from build123d import *

# Parameters (mm, degrees)
SKETCH1_W           = 233.2
SKETCH1_H           = 100
SKETCH1_R           = 1.55
BOSS_EXTRUDE1_DEPTH = 6.35
FILLET1_R           = 5
SKETCH2_R           = 1.55
CUT_EXTRUDE1_DEPTH  = 6.35
SKETCH3_W           = 10
SKETCH3_H           = 12.7
BOSS_EXTRUDE2_DEPTH = 6.35
FILLET2_R           = 5
FILLET3_R           = 10
FILLET4_R           = 2
FILLET5_R           = 20
FILLET6_R           = 5
CUT_EXTRUDE2_DEPTH  = 10
SKETCH5_W           = 120
SKETCH5_H           = 40
CUT_EXTRUDE4_DEPTH  = 10
SKETCH6_R           = 1.5
CUT_EXTRUDE5_DEPTH  = 10
FILLET7_R           = 10
SKETCH7_W           = 25
SKETCH7_H           = 35
CUT_EXTRUDE6_DEPTH  = 10
FILLET9_R           = 10
SKETCH8_R           = 1.5
CUT_EXTRUDE7_DEPTH  = 10
BOSS_EXTRUDE3_START = -6.35
BOSS_EXTRUDE3_DEPTH = 6.35
FILLET10_R          = 5
BOSS_EXTRUDE4_START = -6.35
BOSS_EXTRUDE4_DEPTH = 6.35
FILLET11_R          = 3
FILLET12_R          = 3
CUT_EXTRUDE8_DEPTH  = 10
FILLET13_R          = 3
CUT_EXTRUDE9_DEPTH  = 10
SKETCH13_R          = 1.55
CUT_EXTRUDE10_DEPTH = 10
SKETCH14_R          = 1.5
CUT_EXTRUDE11_DEPTH = 10
BOSS_EXTRUDE5_START = -6.35
BOSS_EXTRUDE5_DEPTH = 6.35
FILLET14_R          = 10
SKETCH15_R          = 1.55
CUT_EXTRUDE12_DEPTH = 254.816001269


# Read off the part's stored shape, not the designer's step: Boss-Extrude5
with BuildPart() as part:
    # Sketch1 → Boss-Extrude1 (new body)
    with BuildSketch(Plane.XY):
        with Locations((116.6, -50)):
            Rectangle(SKETCH1_W, SKETCH1_H)
        with Locations((7.5, -10)):
            Circle(SKETCH1_R, mode=Mode.SUBTRACT)
        with Locations((225.7, -10)):
            Circle(SKETCH1_R, mode=Mode.SUBTRACT)
        with Locations((7.5, -90)):
            Circle(SKETCH1_R, mode=Mode.SUBTRACT)
        with Locations((225.7, -90)):
            Circle(SKETCH1_R, mode=Mode.SUBTRACT)
        with Locations((27.5, -10)):
            Circle(SKETCH1_R, mode=Mode.SUBTRACT)
        with Locations((205.7, -10)):
            Circle(SKETCH1_R, mode=Mode.SUBTRACT)
        with Locations((134.6, -10)):
            Circle(SKETCH1_R, mode=Mode.SUBTRACT)
        with Locations((98.6, -10)):
            Circle(SKETCH1_R, mode=Mode.SUBTRACT)
    extrude(amount=BOSS_EXTRUDE1_DEPTH)

    # Fillet1
    fillet1_edges = [part.edges().sort_by_distance(p)[0] for p in [
        (233.2, -100, 3.175),
        (0, -100, 3.175),
        (0, 0, 3.175),
        (233.2, 0, 3.175),
    ]]
    fillet(fillet1_edges, radius=FILLET1_R)

    # Sketch2 → Cut-Extrude1 (cut)
    with BuildSketch(Plane.XY.offset(6.35)):
        with Locations((45, -25)):
            Circle(SKETCH2_R)
        with Locations((45, -49)):
            Circle(SKETCH2_R)
        with Locations(Location((188.2, -49, 0), (0, 0, 180))):
            Circle(SKETCH2_R)
        with Locations(Location((188.2, -25, 0), (0, 0, 180))):
            Circle(SKETCH2_R)
    extrude(amount=-CUT_EXTRUDE1_DEPTH, mode=Mode.SUBTRACT)

    # Sketch3 → Boss-Extrude2 (add)
    with BuildSketch(Plane.XY.offset(6.35)):
        with Locations((125.723568259, 6.35)):
            Rectangle(SKETCH3_W, SKETCH3_H)
        Polygon((120.723568259, 16.7), (120.723568259, 12.7), (130.723568259, 12.7), (130.723568259, 24.7), (85.723568259, 24.7), (85.723568259, 12.7), (95.723568259, 12.7), (95.723568259, 16.7), align=None)
        Polygon((130.723568259, 12.7), (130.723568259, 0), (152.313568259, 0), (130.723568259, 24.7), align=None)
    extrude(amount=-BOSS_EXTRUDE2_DEPTH)

    # Fillet2
    fillet2_edges = [part.edges().sort_by_distance(p)[0] for p in [
        (85.723568259, 12.7, 3.175),
    ]]
    fillet(fillet2_edges, radius=FILLET2_R)

    # Fillet3
    fillet3_edges = [part.edges().sort_by_distance(p)[0] for p in [
        (120.723568259, 0, 3.175),
    ]]
    fillet(fillet3_edges, radius=FILLET3_R)

    # Fillet4
    fillet4_edges = [part.edges().sort_by_distance(p)[0] for p in [
        (85.723568259, 24.7, 3.175),
    ]]
    fillet(fillet4_edges, radius=FILLET4_R)

    # Fillet5
    fillet5_edges = [part.edges().sort_by_distance(p)[0] for p in [
        (130.723568259, 24.7, 3.175),
        (152.313568259, 0, 3.175),
    ]]
    fillet(fillet5_edges, radius=FILLET5_R)

    # Fillet6
    fillet6_edges = [part.edges().sort_by_distance(p)[0] for p in [
        (120.723568259, 16.7, 3.175),
    ]]
    fillet(fillet6_edges, radius=FILLET6_R)

    # Sketch4 → Cut-Extrude2 (cut)
    with BuildSketch(Plane(origin=(0, 0, 0), x_dir=(-1, 0, 0), z_dir=(0, 0, -1))):
        with BuildLine():
            Line((-110.723568259, 0), (-161.395157905, 0))
            ThreePointArc((-161.395157905, 0), (-153.126132222, 1.789475179), (-146.33682816, 6.837678575))
            Line((-146.33682816, 6.837678575), (-136.700308357, 17.862321425))
            ThreePointArc((-136.700308357, 17.862321425), (-129.911004296, 22.910524821), (-121.641978613, 24.7))
            Line((-121.641978613, 24.7), (-87.723568259, 24.7))
            ThreePointArc((-87.723568259, 24.7), (-86.309354696, 24.114213562), (-85.723568259, 22.7))
            Line((-85.723568259, 22.7), (-85.723568259, 17.7))
            ThreePointArc((-85.723568259, 17.7), (-87.188034353, 14.164466094), (-90.723568259, 12.7))
            Line((-90.723568259, 12.7), (-95.723568259, 12.7))
            Line((-95.723568259, 12.7), (-95.723568259, 16.7))
            Line((-95.723568259, 16.7), (-115.723568259, 16.7))
            ThreePointArc((-115.723568259, 16.7), (-119.259102165, 15.235533906), (-120.723568259, 11.7))
            Line((-120.723568259, 11.7), (-120.723568259, 10))
            ThreePointArc((-120.723568259, 10), (-117.794636071, 2.928932188), (-110.723568259, 0))
        make_face()
    extrude(amount=-CUT_EXTRUDE2_DEPTH, mode=Mode.SUBTRACT)

    # Sketch5 → Cut-Extrude4 (cut)
    with BuildSketch(Plane.XY.offset(6.35)):
        Polygon((56.6, -100), (56.6, -60), (26.6, -100), align=None)
        with Locations((116.6, -80)):
            Rectangle(SKETCH5_W, SKETCH5_H)
        Polygon((206.6, -100), (176.6, -60), (176.6, -100), align=None)
    extrude(amount=-CUT_EXTRUDE4_DEPTH, mode=Mode.SUBTRACT)

    # Sketch6 → Cut-Extrude5 (cut)
    with BuildSketch(Plane.XY.offset(6.35)):
        with Locations((71.6, -21.25)):
            Circle(SKETCH6_R)
        with Locations((161.6, -21.25)):
            Circle(SKETCH6_R)
        with Locations((161.6, -52.75)):
            Circle(SKETCH6_R)
        with Locations((71.6, -52.75)):
            Circle(SKETCH6_R)
    extrude(amount=-CUT_EXTRUDE5_DEPTH, mode=Mode.SUBTRACT)

    # Fillet7
    fillet7_edges = [part.edges().sort_by_distance(p)[0] for p in [
        (206.6, -100, 3.175),
        (26.6, -100, 3.175),
        (56.6, -60, 3.175),
        (176.6, -60, 3.175),
    ]]
    fillet(fillet7_edges, radius=FILLET7_R)

    # Sketch7 → Cut-Extrude6 (cut)
    with BuildSketch(Plane.XY.offset(6.35)):
        Polygon((96.1, -60), (104.1, -60), (104.1, -25), align=None)
        Polygon((129.1, -25), (129.1, -60), (137.1, -60), align=None)
        with Locations((116.6, -42.5)):
            Rectangle(SKETCH7_W, SKETCH7_H)
    extrude(amount=-CUT_EXTRUDE6_DEPTH, mode=Mode.SUBTRACT)

    # Fillet9
    fillet9_edges = [part.edges().sort_by_distance(p)[0] for p in [
        (137.1, -60, 3.175),
        (96.1, -60, 3.175),
        (104.1, -25, 3.175),
        (129.1, -25, 3.175),
    ]]
    fillet(fillet9_edges, radius=FILLET9_R)

    # Sketch8 → Cut-Extrude7 (cut)
    with BuildSketch(Plane.XY.offset(6.35)):
        with Locations((53.6, -21.25)):
            Circle(SKETCH8_R)
    extrude(amount=-CUT_EXTRUDE7_DEPTH, mode=Mode.SUBTRACT)

    # Sketch9 → Boss-Extrude3 (add)
    with BuildSketch(Plane.XY.offset(6.35).offset(BOSS_EXTRUDE3_START)):
        with BuildLine():
            Line((53.6, -64), (52.97582451, -64.832233986))
            Line((52.97582451, -64.832233986), (80.428117061, -87.022837132))
            ThreePointArc((80.428117061, -87.022837132), (90.975638571, -85.904897064), (89.857698503, -75.357375554))
            Line((89.857698503, -75.357375554), (70.858883385, -60))
            Line((70.858883385, -60), (61.6, -60))
            ThreePointArc((61.6, -60), (57.127864045, -61.05572809), (53.6, -64))
        make_face()
        with BuildLine():
            ThreePointArc((83.976361625, -80.247148199), (85.642998156, -79.775924736), (86.642907782, -81.190106343))
            ThreePointArc((86.642907782, -81.190106343), (84.642817409, -82.60428795), (83.976361625, -80.247148199))
        make_face(mode=Mode.SUBTRACT)
    boss_extrude3 = extrude(amount=BOSS_EXTRUDE3_DEPTH)

    # Mirror1: Boss-Extrude3 across plane
    add(boss_extrude3.mirror(Plane.ZY.offset(-116.6)))

    # Fillet10
    fillet10_edges = [part.edges().sort_by_distance(p)[0] for p in [
        (52.97582451, -64.832233986, 3.175),
        (70.858883385, -60, 3.175),
        (180.22417549, -64.832233986, 3.175),
        (162.341116615, -60, 3.175),
    ]]
    fillet(fillet10_edges, radius=FILLET10_R)

    # Sketch10 → Boss-Extrude4 (add)
    with BuildSketch(Plane.XY.offset(6.35).offset(BOSS_EXTRUDE4_START)):
        with BuildLine():
            ThreePointArc((29.6, -96), (26.844092638, -98.514663376), (23.358283237, -99.844208453))
            Line((23.358283237, -99.844208453), (86.46162021, -88.573262682))
            ThreePointArc((86.46162021, -88.573262682), (83.276282006, -88.454107183), (80.428117061, -87.022837132))
            Line((80.428117061, -87.022837132), (72.798322589, -80.855419933))
            Line((72.798322589, -80.855419933), (36.033483436, -87.422022085))
            Line((36.033483436, -87.422022085), (29.6, -96))
        make_face()
    boss_extrude4 = extrude(amount=BOSS_EXTRUDE4_DEPTH)

    # Fillet11
    fillet11_edges = [part.edges().sort_by_distance(p)[0] for p in [
        (36.033483436, -87.422022085, 3.175),
        (72.798322589, -80.855419933, 3.175),
    ]]
    fillet(fillet11_edges, radius=FILLET11_R)

    # Mirror3: Boss-Extrude4 across plane
    add(boss_extrude4.mirror(Plane.ZY.offset(-116.6)))

    # Fillet12
    fillet12_edges = [part.edges().sort_by_distance(p)[0] for p in [
        (197.166516564, -87.422022085, 3.175),
        (160.401677411, -80.855419933, 3.175),
    ]]
    fillet(fillet12_edges, radius=FILLET12_R)

    # Sketch11 → Cut-Extrude8 (cut)
    with BuildSketch(Plane.XY.offset(6.35)):
        Polygon((35.5, -50), (18, -82), (18, -18), align=None)
        Polygon((215.2, -18), (215.2, -82), (197.7, -50), align=None)
    extrude(amount=-CUT_EXTRUDE8_DEPTH, mode=Mode.SUBTRACT)

    # Fillet13
    fillet13_edges = [part.edges().sort_by_distance(p)[0] for p in [
        (35.5, -50, 3.175),
        (18, -82, 3.175),
        (18, -18, 3.175),
        (215.2, -18, 3.175),
        (215.2, -82, 3.175),
        (197.7, -50, 3.175),
    ]]
    fillet(fillet13_edges, radius=FILLET13_R)

    # Sketch12 → Cut-Extrude9 (cut)
    with BuildSketch(Plane.XY.offset(6.35)):
        with BuildLine():
            ThreePointArc((186.5, -65), (188.2, -66.7), (189.9, -65))
            ThreePointArc((189.9, -65), (188.2, -63.3), (186.5, -65))
        make_face()
        with BuildLine():
            ThreePointArc((43.3, -65), (45, -66.7), (46.7, -65))
            ThreePointArc((46.7, -65), (45, -63.3), (43.3, -65))
        make_face()
    extrude(amount=-CUT_EXTRUDE9_DEPTH, mode=Mode.SUBTRACT)

    # Sketch13 → Cut-Extrude10 (cut)
    with BuildSketch(Plane.XY.offset(6.35)):
        with Locations((161.599999999, -84.25)):
            Circle(SKETCH13_R)
        with Locations((71.6, -84.25)):
            Circle(SKETCH13_R)
    extrude(amount=-CUT_EXTRUDE10_DEPTH, mode=Mode.SUBTRACT)

    # Sketch14 → Cut-Extrude11 (cut)
    with BuildSketch(Plane(origin=(0, 0, 0), x_dir=(-1, 0, 0), z_dir=(0, 0, -1))):
        with Locations((-22.5, -90)):
            Circle(SKETCH14_R)
        with Locations((-35, -90)):
            Circle(SKETCH14_R)
        with Locations((-47.5, -90)):
            Circle(SKETCH14_R)
    extrude(amount=-CUT_EXTRUDE11_DEPTH, mode=Mode.SUBTRACT)

    # Boss-Extrude5 outline → Boss-Extrude5 (add)
    with BuildSketch(Plane(origin=(0, 0, 0), x_dir=(-1, 0, 0), z_dir=(0, 0, -1)).offset(BOSS_EXTRUDE5_START)):
        with BuildLine():
            Line((-87.900343264, -88.164814191), (-58.358283237, -99.844208453))
            Line((-58.358283237, -99.844208453), (-21.684763887, -99.999640748))
            ThreePointArc((-21.684763887, -99.999640748), (-22.524794828, -99.957145902), (-23.358283237, -99.844208453))
            Line((-23.358283237, -99.844208453), (-86.46162021, -88.573262682))
            ThreePointArc((-86.46162021, -88.573262682), (-87.191188278, -88.404990057), (-87.900343264, -88.164814191))
        make_face()
    extrude(amount=BOSS_EXTRUDE5_DEPTH)

    # Fillet14
    fillet14_edges = [part.edges().sort_by_distance(p)[0] for p in [
        (58.358283237, -99.844208453, 3.175),
    ]]
    fillet(fillet14_edges, radius=FILLET14_R)

    # Sketch15 → Cut-Extrude12 (cut, through all)
    with BuildSketch(Plane(origin=(0, 0, 0), x_dir=(-1, 0, 0), z_dir=(0, 0, -1))):
        with Locations((-179.6, -21.25)):
            Circle(SKETCH15_R)
    extrude(amount=-CUT_EXTRUDE12_DEPTH, mode=Mode.SUBTRACT)


solid = part.part
Geometry: final body of the model. Coordinates: model frame, mm. A direction names the side the tool comes from. Coordinates: 2 decimals unless noted, no trailing zeros. Write each loop counter-clockwise with the first axis right and the second up, starting at its lowest first coordinate (ties: lowest second). Pieces come first, ordered by that corner, then holes. Notation, with made-up numbers: (26, 14) - (74, 14) arc R19 ccw to (74, 39) - close; hole circle Ø8 at (54, -14). An arc over 180 degrees is marked (long way). Return JSON: item names as keys, results as strings.
Item 1: Section query B-B (z = 1.5). Count the separate pieces of the cut face and the enclosed holes in it, and give its area (3 significant figures).
Completed:
{"separate pieces": "1", "enclosed holes": "31", "area": "17,300 mm2"}
Item 2: Pull-direction query (X, two-part tool) for faces 4 (the face through (233.2, -51, 3)), 5 (the face through (138.912, -57.878, 3.131)), 6 (the face through (13, -100, 3)); classes: +X half, -X half, draft (parallel to the pull), parting line (faces both ways), or undercut.
Completed:
{"face 4": "+X half", "face 5": "undercut", "face 6": "draft"}
Item 3: Line query: L1, parallel to X at y = -61, z = 4.5; L2, parallel to X at y = -28.5, z = 4.5; L3, parallel to X at y = -52.5, z = 5. Output: solid intervals per line, ascending.
Completed:
{"L1": "x = 0 to 18, 29.48 to 82, 151.2 to 203.72, 215.2 to 233.2", "L2": "x = 0 to 18.27, 23.74 to 104.47, 128.73 to 209.46, 214.93 to 233.2", "L3": "x = 0 to 18, 34.13 to 70.12, 73.08 to 97.81, 135.39 to 160.12, 163.08 to 199.07, 215.2 to 233.2"}
Item 4: Reachability of faces 1 (the face through (220, -100, 3)), 2 (the face through (127.435, -27.24, 3.131)), 3 (the face through (29.25, -61.43, 3.22)) from +Z, -Z, +X, -X, +Y, -Y: full face, straight path, thin tool, end or side. Return the list, or none.
Completed:
{"face 1": "+Z, -Z, +X, -X, -Y", "face 2": "+Z, -Z, -Y", "face 3": "+Z, -Z"}
Item 5: Section query A-A (y = -38.5). Output: boundary loops of the cut face in (x, z), and give its area (3 significant figures).
Completed:
{"outline": "(0, 0) - (18, 0) - (18, 6.35) - (0, 6.35) - close; (29.21, 0) - (101.01, 0) - (101.01, 6.35) - (29.21, 6.35) - close; (132.19, 0) - (203.99, 0) - (203.99, 6.35) - (132.19, 6.35) - close; (215.2, 0) - (233.2, 0) - (233.2, 6.35) - (215.2, 6.35) - close", "area": "1,140 mm2"}
Item 6: Section query C-C (x = 115). Output: boundary loops of the cut face in (y, z).
Completed:
{"outline": "(-25, 0) - (0, 0) - (0, 6.35) - (-25, 6.35) - close"}
